```python
from build123d import *

# Parameters (mm, degrees)
F0_R     = 3.4
F0_R_2   = 1.9
F1_DEPTH = 10
F0_R_3   = 2
F2_DEPTH = 2


with BuildPart() as f1:
    # F0 (on Top) → F1 (new body)
    with BuildSketch(Plane.XY):
        with Locations((0, 4)):
            Circle(F0_R)
        with Locations((0, 4)):
            Circle(F0_R_2, mode=Mode.SUBTRACT)
    extrude(amount=F1_DEPTH)

    # F0 (on Top) → F2 (join)
    with BuildSketch(Plane.XY):
        with BuildLine():
            ThreePointArc((-5, 4), (-3.535534, 0.464466), (0, -1))
            ThreePointArc((0, -1), (3.535534, 0.464466), (5, 4))
            ThreePointArc((5, 4), (0, 9), (-5, 4))
        make_face()
        with Locations((0, 4)):
            Circle(F0_R, mode=Mode.SUBTRACT)
        with BuildLine():
            ThreePointArc((0, -1), (3.535534, -2.464466), (5, -6))
            Line((5, -6), (5, 4))
            ThreePointArc((5, 4), (3.535534, 0.464466), (0, -1))
        make_face()
        with BuildLine():
            ThreePointArc((0, -1), (-3.535534, -2.464466), (-5, -6))
            ThreePointArc((-5, -6), (0, -11), (5, -6))
            ThreePointArc((5, -6), (3.535534, -2.464466), (0, -1))
        make_face()
        with Locations((0, -6)):
            Circle(F0_R_3, mode=Mode.SUBTRACT)
        with BuildLine():
            Line((-5, 4), (-5, -6))
            ThreePointArc((-5, -6), (-3.535534, -2.464466), (0, -1))
            ThreePointArc((0, -1), (-3.535534, 0.464466), (-5, 4))
        make_face()
    extrude(amount=F2_DEPTH)


solid = f1.part
```
Design review of the part built by this model. Coordinates are the model's own, in mm. A direction names the side the tool comes from. Round coordinates to 2 decimals unless told otherwise and drop trailing zeros. Order: outer loops, then holes, each group sorted by start corner. A loop starts at its lowest first (then second) coordinate and runs counter-clockwise, first axis right, second up. Notation, with made-up numbers: M 84.5,-29 L 137.5,-29 A36 ccw 137.5,6 Z; hole C -13.75,4 d6. An arc over 180 degrees is marked long. Put each result on its own line as item: value.
Q1. Consider section B-B (y = -4.5). State the section outline as (x, z) points.
Reported:
outline: M -5,0 L -1.32,0 L -1.32,2 L -5,2 Z; M 1.32,0 L 5,0 L 5,2 L 1.32,2 Z
Q2. Consider section A-A (x = 0). State the section outline as (y, z) points, and give its area (3 significant figures).
Reported:
outline: M -11,0 L -8,0 L -8,2 L -11,2 Z; M -4,0 L 2.1,0 L 2.1,10 L 0.6,10 L 0.6,2 L -4,2 Z; M 5.9,0 L 9,0 L 9,2 L 7.4,2 L 7.4,10 L 5.9,10 Z
area: 48.4 mm²
Q3. Consider section D-D (x = -3). State the section outline as (y, z) points.
Reported:
outline: M -10,0 L 8,0 L 8,2 L 5.6,2 L 5.6,10 L 2.4,10 L 2.4,2 L -10,2 Z
Q4. Consider section C-C (z = 5.25). State the section outline as (x, y) points, and give its area (3 significant figures).
Reported:
outline: C 0,4 d6.8; hole C 0,4 d3.8
area: 25.0 mm²
Q5. To check wall thickness, follow line 1 (Y direction, x = 0, z = 0.7); line 2 (Y direction, x = 0, z = 5.25); line 3 (Y direction, x = -1, z = 1.5). State the ranges of each line that lie inside material, in increasing order.
Reported:
line 1: -11 to -8, -4 to 2.1, 5.9 to 9
line 2: 0.6 to 2.1, 5.9 to 7.4
line 3: -10.9 to -7.73, -4.27 to 2.38, 5.62 to 8.9
Q6. Draft analysis for pull direction X (two halves, no side actions). For faces 3 (the face through (5, -1, 1)), 4 (the face through (-0.247, 5.884, 4.93)), 5 (the face through (0, 9, 1)), state which applies: released by +X, released by -X, zero draft, split by the parting line, or undercut.
Reported:
face 3: released by +X
face 4: undercut
face 5: split by the parting line
Q7. Insertion check: pin 1 Ø1 at (x, z) = (-1, 5.5) entering from +Y; pin 2 Ø1 at (x, z) = (3, 2) entering from +Y; pin 3 Ø1.5 at (y, z) = (4.5, 9) entering from -X. Each pin has a flat end and moves straight along its axis. Give the tip position at first contact, or say it passes through.
Reported:
pin 1: y = 7.36
pin 2: y = 8.33
pin 3: x = -3.4
Q8. Machinability: for faces 1 (the face through (0, -1, 0)), 2 (the face through (-2.506, 6.298, 5.944)), which of the approach directions +Z, -Z, +X, -X, +Y, -Y give a long, thin tool a straight path to every point of the face, cutting with its end or side? Answer none if there is none.
Reported:
face 1: -Z, +X, -X, +Y, -Y
face 2: +Z
